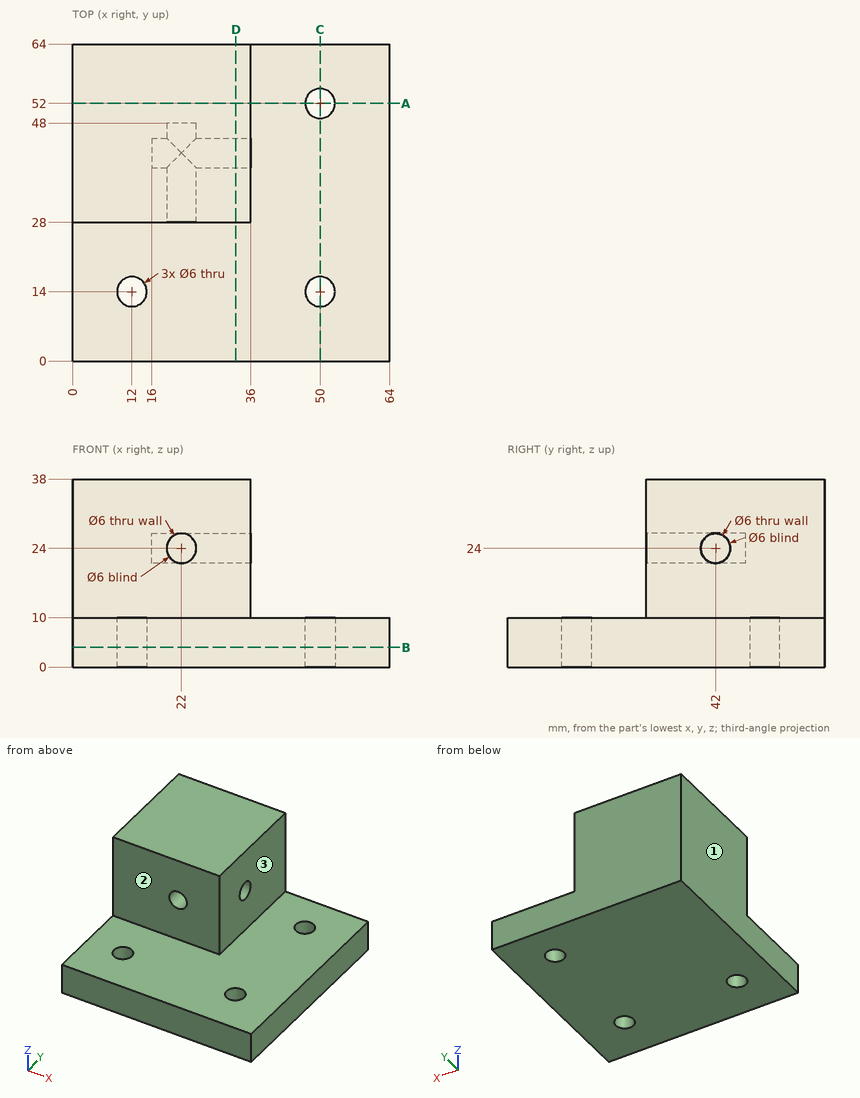
Source: three-view drawing plus pictorial views. Frame: mm from the lowest corner of the part. A direction names the side the tool comes from. Coordinates: 2 decimals unless noted, no trailing zeros. Order: outer loops, then holes, each group sorted by start corner. A loop starts at its lowest first (then second) coordinate and runs counter-clockwise, first axis right, second up. Notation, with made-up numbers: M 12.5,34.25 L 18.5,34.25 A29 ccw 18.5,68.25 Z; hole C -12.5,34 d3. An arc over 180 degrees is marked long. One line per question, with ' | ' between items.
Item 1: Section A-A (y = 52). Output: boundary loops of the cut face in (x, z).
Geometry results:
outline: M 0,0 L 47,0 L 47,10 L 36,10 L 36,38 L 0,38 Z; M 53,0 L 64,0 L 64,10 L 53,10 Z
Item 2: Ray query, line 1 along Y through (x, z) = (50, 6); line 2 along Z through (x, y) = (22, 46.2); line 3 along X through (y, z) = (12, 5). Return the intervals inside material, ascending.
Geometry results:
line 1: y = 0 to 11, 17 to 49, 55 to 64 | line 2: z = 0 to 21, 27 to 38 | line 3: x = 0 to 9.76, 14.24 to 47.76, 52.24 to 64
Item 3: Section B-B (z = 4). Output: boundary loops of the cut face in (x, y), then the cut area to 3 significant figures.
Geometry results:
outline: M 0,0 L 64,0 L 64,64 L 0,64 Z; hole C 12,14 d6; hole C 50,14 d6; hole C 50,52 d6 | area: 4,010 mm^2
Item 4: Pin query (flat end, axial travel): pin 1 (8 mm diameter, centred on x = 27, y = 18.5, fed in from +Z); pin 2 (12 mm diameter, centred on y = 43, z = 20.5, fed in from +X); pin 3 (5 mm diameter, centred on x = 12, y = 14, fed in from +Z); pin 4 (3.5 mm diameter, centred on y = 42, z = 24, fed in from +X). Return the tip coordinate at first contact, or that it passes through.
Geometry results:
pin 1: stops at z = 10 | pin 2: stops at x = 36 | pin 3: passes through | pin 4: stops at x = 16
Item 5: Reachability of the marked faces 1, 2 and 3 from +Z, -Z, +X, -X, +Y, -Y: full face, straight path, thin tool, end or side. Return the list, or none.
Geometry results:
face 1: +Z, -Z, -X, +Y, -Y | face 2: +Z, +X, -X, -Y | face 3: +Z, +X, +Y, -Y
Item 6: Section D-D (x = 33). Output: boundary loops of the cut face in (y, z).
Geometry results:
outline: M 0,0 L 64,0 L 64,38 L 28,38 L 28,10 L 0,10 Z; hole C 42,24 d6
Item 7: Section C-C (x = 50). Output: boundary loops of the cut face in (y, z), then the cut area to 3 significant figures.
Geometry results:
outline: M 0,0 L 11,0 L 11,10 L 0,10 Z; M 17,0 L 49,0 L 49,10 L 17,10 Z; M 55,0 L 64,0 L 64,10 L 55,10 Z | area: 520 mm^2
